from build123d import *

# Parameters (mm, degrees)
F0_W     = 203.2
F0_H     = 304.8
F1_DEPTH = 6.35
F2_W     = 12.7
F2_H     = 304.8
F2_W_2   = 88.9
F2_W_3   = 25.4
F2_H_2   = 203.2
F3_DEPTH = 12.7
F4_W     = 88.9
F4_H     = 304.8
F4_W_2   = 25.4
F4_H_2   = 203.2
F4_W_3   = 12.7
F5_DEPTH = 12.7
F6_W     = 203.2
F6_H     = 88.9
F6_R     = 12.7
F7_DEPTH = 12.7
F8_SIZE  = 0.508
F9_SIZE  = 25.4


with BuildPart() as f1:
    # F0 (on Front) → F1 (new body, symmetric)
    with BuildSketch(Plane.XZ):
        Rectangle(F0_W, F0_H)
    extrude(amount=F1_DEPTH, both=True)

    # F2 (on face) → F3 (join)
    with BuildSketch(Plane.YZ.offset(101.6)):
        Rectangle(F2_W, F2_H)
        with Locations((-50.8, 0)):
            Rectangle(F2_W_2, F2_H)
        with Locations((-57.15, 0)):
            Rectangle(F2_W_3, F2_H_2, mode=Mode.SUBTRACT)
    extrude(amount=F3_DEPTH)

    # F4 (on face) → F5 (join)
    with BuildSketch(Plane(origin=(-101.6, 0, 0), x_dir=(0, -1, 0), z_dir=(-1, 0, 0))):
        with Locations((50.8, 0)):
            Rectangle(F4_W, F4_H)
        with Locations((57.15, 0)):
            Rectangle(F4_W_2, F4_H_2, mode=Mode.SUBTRACT)
        Rectangle(F4_W_3, F4_H)
    extrude(amount=F5_DEPTH)

    # F6 (on face) → F7 (join)
    with BuildSketch(Plane.XY.offset(152.4)):
        with Locations((0, -50.8)):
            Rectangle(F6_W, F6_H)
        with Locations((0, -31.75)):
            Circle(F6_R, mode=Mode.SUBTRACT)
    extrude(amount=-F7_DEPTH)

    # F8
    f8_edges = [f1.edges().sort_by_distance(p)[0] for p in [
        (-12.7, -31.75, 152.4),
        (-12.7, -31.75, 139.7),
    ]]
    chamfer(f8_edges, length=F8_SIZE)

    # F9
    f9_edges = [f1.edges().sort_by_distance(p)[0] for p in [
        (107.95, -95.25, -152.4),
        (-107.95, -95.25, -152.4),
    ]]
    chamfer(f9_edges, length=F9_SIZE)


solid = f1.part
Build history of the part. All positions in model axes, mm. A direction names the side the tool comes from. Give positions to 0.01 mm unless a question says otherwise; leave off trailing zeros. Write each loop counter-clockwise with the first axis right and the second up, starting at its lowest first coordinate (ties: lowest second). Pieces come first, ordered by that corner, then holes. Notation, with made-up numbers: (-19, 81.25) - (-6, 81.25) arc R17 ccw to (-6, 104.25) - close; hole circle Ø8 at (-35, -21). An arc over 180 degrees is marked (long way). Use one line per item in the form item = value. Start each with the question number.
1. Drop flat-ended pins along their axis: pin 1 Ø12 at (x, y) = (63, -56.5) entering from -Z; pin 2 Ø15 at (x, y) = (0, -31.75) entering from +Z. Give the stop position or say it passes through.
2. Probe line 1 (X direction, y = -8, z = 133.5); line 2 (X direction, y = -31, z = 145); line 3 (Y direction, x = 0, z = 145.25). List the from-to ranges inside material, lowest first. Write a range as [from, to].
3. Two-plate mould, pull along Z, no slides. Class faces 1 (the face through (-108, -69.85, -1)), 2 (the face through (-108, -57, -101.6)), 3 (the face through (-101.6, -40, -4)), 4 (the face through (-2, -55, 152.4)): released by +Z, released by -Z, zero draft, split by the parting line, or undercut.
4. Band-saw the part on B-B on y = -31.75. Write the cut outline in (x, z), plus the area to 4 significant figures.
5. Band-saw the part on D-D on z = -106.5. Write the cut outline in (x, y), plus the area to 3 significant figures.
6. Band-saw the part on A-A on z = 5. Write the cut outline in (x, y).
7. 3-axis set-ups, long thin cutter, end or side, ignore diameter. For faces 5 (the face through (-108, -44.45, -1)), 6 (the face through (114.3, -34, 2)), 7 (the face through (-1, -6.35, -4)): which of +Z, -Z, +X, -X, +Y, -Y reach the whole face in a straight line?
8. Band-saw the part on C-C on x = 0. Write the cut outline in (y, z).
Conclusion:
q1.pin_1 = 139.7
q1.pin_2 = through
q2.line_1 = [-114.3, -101.6], [101.6, 114.3]
q2.line_2 = [-114.3, -12.68], [12.68, 114.3]
q2.line_3 = [-95.25, -44.45], [-19.05, 6.35]
q3.face_1 = undercut
q3.face_2 = undercut
q3.face_3 = zero draft
q3.face_4 = released by +Z
q4.outline = (-114.3, -152.4) - (-101.6, -152.4) - (-101.6, 139.7) - (-13.21, 139.7) - (-12.7, 140.21) - (-12.7, 151.89) - (-13.21, 152.4) - (-114.3, 152.4) - close; (12.7, 140.21) - (13.21, 139.7) - (101.6, 139.7) - (101.6, -152.4) - (114.3, -152.4) - (114.3, 152.4) - (13.21, 152.4) - (12.7, 151.89) - close
q4.area = 10,000 mm²
q5.outline = (-114.3, -95.25) - (-101.6, -95.25) - (-101.6, -6.35) - (101.6, -6.35) - (101.6, -95.25) - (114.3, -95.25) - (114.3, 6.35) - (-114.3, 6.35) - close
q5.area = 5,160 mm²
q6.outline = (-114.3, -95.25) - (-101.6, -95.25) - (-101.6, -69.85) - (-114.3, -69.85) - close; (-114.3, -44.45) - (-101.6, -44.45) - (-101.6, -6.35) - (101.6, -6.35) - (101.6, -44.45) - (114.3, -44.45) - (114.3, 6.35) - (-114.3, 6.35) - close; (101.6, -95.25) - (114.3, -95.25) - (114.3, -69.85) - (101.6, -69.85) - close
q7.face_5 = +X, -X
q7.face_6 = +Z, -Z, +X, +Y, -Y
q7.face_7 = -Z, -Y
q8.outline = (-95.25, 139.7) - (-44.96, 139.7) - (-44.45, 140.21) - (-44.45, 151.89) - (-44.96, 152.4) - (-95.25, 152.4) - close; (-19.05, 140.21) - (-18.54, 139.7) - (-6.35, 139.7) - (-6.35, -152.4) - (6.35, -152.4) - (6.35, 152.4) - (-18.54, 152.4) - (-19.05, 151.89) - close
